Input: part model. Units: mm. Frame: model coordinates. Face numbers are marked on the shaded views. A direction names the side the tool comes from. Coordinates: 2 decimals unless noted, no trailing zeros. Loops run counter-clockwise (first coordinate to the right, second up) from the corner with the lowest first, then second, coordinate; pieces in that order, holes last. Notation, with made-up numbers: (54.25, 87) -> (95.25, 87) arc R17 cw to (95.25, 104) -> close; hole circle Ø11 at (-26.75, 28). An arc over 180 degrees is marked (long way). Put each result on its own line as item: value. Start each with the question number.
1) Set-up query: the marked faces 1 and 2. Return all of +Z, -Z, +X, -X, +Y, -Y with unobstructed straight access to the full face (end or side cutting, diameter ignored); none if empty.
2) Cut plane D-D (x = 15.5). Return the cut outline in (y, z).
3) Pull-direction query (Z, two-part tool) for the marked faces 3, 4, 5 and 6; classes: pulls with the +Z half, pulls with the -Z half, needs draft (parallel to the pull), parting line crosses it, or undercut.
4) Cut plane A-A (z = 15.5). Return the cut outline in (x, y).
5) Cut plane B-B (y = 10.8). State how many separate pieces and enclosed holes the cut face has, plus the area to 3 significant figures.
6) Material intervals for L1, parallel to X at y = 1, z = 28; L2, parallel to X at y = 6.5, z = 29 (3 decimals); L3, parallel to Z at x = 14.5, y = 1, sorted ascending.
7) Contact query for a flat-ended pin moving along its axis: P1, Ø8, axis at x = 16.5, y = 14.5, coming from the -Z side. Output: stop coordinate, or through.
8) Cut plane C-C (x = 1.5). Return the cut outline in (y, z), plus the area to 3 significant figures.
from build123d import *

# Parameters (mm, degrees)
BOSS_EXTRUDE1_DEPTH = 21.6
SKETCH4_R           = 1.75
SKETCH4_W           = 22.75
SKETCH4_H           = 11.6
CUT_EXTRUDE2_DEPTH  = 50


with BuildPart() as part:
    # Sketch2 → Boss-Extrude1 (new body)
    with BuildSketch(Plane(origin=(0, 0, 0), x_dir=(1, 0, 0), z_dir=(0, 1, 0))):
        Polygon((-22.5, 0), (22.5, 0), (22.5, -30.48), (10.5, -30.48), (10.5, -28.89), (20.91, -28.89), (20.91, -1.59), (-20.91, -1.59), (-20.91, -28.89), (-10.5, -28.89), (-10.5, -30.48), (-22.5, -30.48), align=None)
    extrude(amount=BOSS_EXTRUDE1_DEPTH)

    # Sketch4 → Cut-Extrude2 (cut)
    with BuildSketch(Plane(origin=(0, 0, 0), x_dir=(-1, 0, 0), z_dir=(0, 0, -1))):
        with Locations((-14.875, 10.8)):
            Circle(SKETCH4_R)
        with Locations((14.875, 10.8)):
            Circle(SKETCH4_R)
        with Locations((0, 10.8)):
            Rectangle(SKETCH4_W, SKETCH4_H)
    extrude(amount=-CUT_EXTRUDE2_DEPTH, mode=Mode.SUBTRACT)


solid = part.part
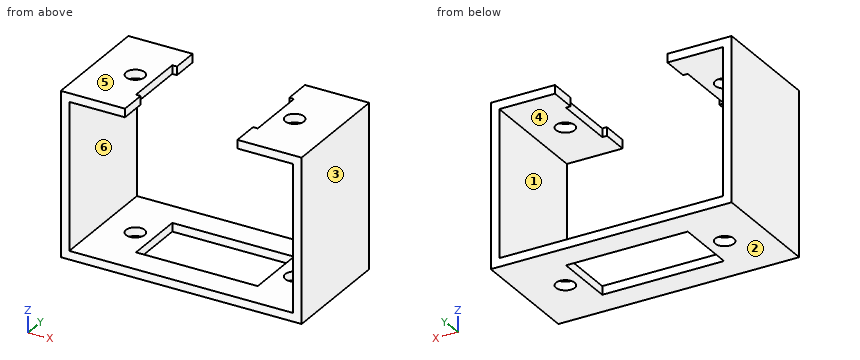
Results found:
1. face 1: +Y, -Y
1. face 2: -Z, +X, -X, +Y, -Y
2. outline: (0, 0) -> (9.17, 0) -> (9.17, 1.59) -> (0, 1.59) -> close; (0, 28.89) -> (9.17, 28.89) -> (9.17, 30.48) -> (0, 30.48) -> close; (12.43, 0) -> (21.6, 0) -> (21.6, 1.59) -> (12.43, 1.59) -> close; (12.43, 28.89) -> (21.6, 28.89) -> (21.6, 30.48) -> (12.43, 30.48) -> close
3. face 3: needs draft
3. face 4: undercut
3. face 5: pulls with the +Z half
3. face 6: undercut
4. outline: (-22.5, 0) -> (-20.91, 0) -> (-20.91, 21.6) -> (-22.5, 21.6) -> close; (20.91, 0) -> (22.5, 0) -> (22.5, 21.6) -> (20.91, 21.6) -> close
5. separate pieces: 6
5. enclosed holes: 0
5. area: 135 mm2
6. L1: x = -22.5 to -20.91, 20.91 to 22.5
6. L2: x = -22.5 to -11.375, 11.375 to 22.5
6. L3: z = 0 to 1.59, 28.89 to 30.48
7. P1: stops at z = 0
8. outline: (0, 0) -> (5, 0) -> (5, 1.59) -> (0, 1.59) -> close; (16.6, 0) -> (21.6, 0) -> (21.6, 1.59) -> (16.6, 1.59) -> close
8. area: 15.9 mm2
